from build123d import *

# Parameters (mm, degrees)
F0_R     = 15
F1_DEPTH = 50
F3_DEPTH = 50.001
F4_DEPTH = 20
F6_DEPTH = 15


with BuildPart() as f1:
    # F0 (on Top) → F1 (new body)
    with BuildSketch(Plane.XY):
        Circle(F0_R)
    extrude(amount=F1_DEPTH)

    # F2 (on Top) → F3 (cut, through all)
    with BuildSketch(Plane.XY):
        with BuildLine():
            ThreePointArc((6, 0), (4.242641, 4.242641), (0, 6))
            ThreePointArc((0, 6), (-4.242641, 4.242641), (-6, 0))
            ThreePointArc((-6, 0), (-4.242641, -4.242641), (0, -6))
            ThreePointArc((0, -6), (4.242641, -4.242641), (6, 0))
        make_face()
    extrude(amount=F3_DEPTH, mode=Mode.SUBTRACT)

    # F2 (on Top) → F4 (cut)
    with BuildSketch(Plane.XY):
        with BuildLine():
            Line((6, 0), (6, 6))
            Line((6, 6), (0, 6))
            ThreePointArc((0, 6), (4.242641, 4.242641), (6, 0))
        make_face()
        with BuildLine():
            ThreePointArc((-6, 0), (-4.242641, 4.242641), (0, 6))
            Line((0, 6), (-6, 6))
            Line((-6, 6), (-6, 0))
        make_face()
        with BuildLine():
            Line((6, -6), (6, 0))
            ThreePointArc((6, 0), (4.242641, -4.242641), (0, -6))
            Line((0, -6), (6, -6))
        make_face()
        with BuildLine():
            ThreePointArc((0, -6), (-4.242641, -4.242641), (-6, 0))
            Line((-6, 0), (-6, -6))
            Line((-6, -6), (0, -6))
        make_face()
    extrude(amount=F4_DEPTH, mode=Mode.SUBTRACT)

    # F5 (on face) → F6 (cut)
    with BuildSketch(Plane.XY.offset(50)):
        Polygon((9.5, 5.484828), (0, 10.969655), (-9.5, 5.484828), (-9.5, -5.484828), (0, -10.969655), (9.5, -5.484828), align=None)
    extrude(amount=-F6_DEPTH, mode=Mode.SUBTRACT)


solid = f1.part
CAD build for the part. Positions are in the model's coordinates, mm. A direction names the side the tool comes from. Coordinates: 2 decimals unless noted, no trailing zeros. Loops run counter-clockwise (first coordinate to the right, second up) from the corner with the lowest first, then second, coordinate; pieces in that order, holes last. Notation, with made-up numbers: (20.5, 39) - (54.5, 39) arc R30 cw to (54.5, 78) - close; hole circle Ø10 at (37.5, 60). An arc over 180 degrees is marked (long way). Use one line per item in the form item = value. Start each with the question number.
1) Two-plate mould, pull along X, no slides. Class faces 4 (the face through (6.5, 0.2, 0)), 5 (the face through (-4.684, 8.266, 42.605)), 6 (the face through (-14.985, 0.66, 24.65)): +X half, -X half, draft (parallel to the pull), parting line (faces both ways), or undercut.
2) Tool access for faces 1 (the face through (0, -6, 10)), 2 (the face through (10, 0, 50)), 3 (the face through (-4, -5, 35)): list every direction of +Z, -Z, +X, -X, +Y, -Y with a clear straight run to the whole face (end or side of a thin tool).
3) Flat gauge pins, fed straight in: pin 1 (10 mm diameter, centred on x = 10.5, z = 36.5, fed in from +Y); pin 2 (6 mm diameter, centred on x = -4, z = 13.5, fed in from -Y); pin 3 (6 mm diameter, centred on x = -10.5, z = 23, fed in from -Y). Where does each tip first touch, or does it go through?
4) Band-saw the part on B-B (x = 1.75). Give the cut face in (y, z), and give its area (3 significant figures).
5) Band-saw the part on C-C (x = 7.5). Give the cut face in (y, z), and give its area (3 significant figures).
6) Drill centre lines: L1, parallel to Y at x = 2.5, z = 28; L2, parallel to Z at x = -0.5, y = 7; L3, parallel to X at y = -4, z = 27. Where is each one in solid material? Low to high. Write a range as from..to.
7) Band-saw the part on D-D (y = -7.5). Give the cut face in (x, z).
8) Band-saw the part on A-A (z = 4.5). Give the cut face in (x, y).
Check values:
q1.face_4 = draft
q1.face_5 = undercut
q1.face_6 = parting line
q2.face_1 = -Z
q2.face_2 = +Z, +X, -X, +Y, -Y
q2.face_3 = +Z
q3.pin_1 = 13.96
q3.pin_2 = -14.97
q3.pin_3 = -12.99
q4.outline = (-14.9, 0) - (-6, 0) - (-6, 20) - (-5.74, 20) - (-5.74, 35) - (-9.96, 35) - (-9.96, 50) - (-14.9, 50) - close; (5.74, 20) - (6, 20) - (6, 0) - (14.9, 0) - (14.9, 50) - (9.96, 50) - (9.96, 35) - (5.74, 35) - close
q4.area = 779 mm2
q5.outline = (-12.99, 0) - (12.99, 0) - (12.99, 50) - (6.64, 50) - (6.64, 35) - (-6.64, 35) - (-6.64, 50) - (-12.99, 50) - close
q5.area = 1,100 mm2
q6.L1 = -14.79..-5.45, 5.45..14.79
q6.L2 = 0..35
q6.L3 = -14.46..-4.47, 4.47..14.46
q7.outline = (-12.99, 0) - (12.99, 0) - (12.99, 50) - (6.01, 50) - (6.01, 35) - (-6.01, 35) - (-6.01, 50) - (-12.99, 50) - close
q8.outline = circle Ø30 at (0, 0); hole (-6, -6) - (6, -6) - (6, 6) - (-6, 6) - close
